The listing builds one solid part. Answer for the finished solid, in the listing's coordinates (mm). Give positions to 0.01 mm unless a question says otherwise; leave off trailing zeros. Answer as CSV lines item,"result". Start each with the question number.
(1) Each of these flat-tipped pins is pushed along its axis until it touches: pin 1 Ø10 at (x, y) = (89.5, -16.5) entering from -Z; pin 2 Ø1.6 at (x, z) = (107, 1) entering from -Y; pin 3 Ø1.5 at (x, z) = (129.5, 0.5) entering from -Y. Where does it stop, or does it pass through?
(2) Straight lines are drawn through the part: probe 1 along X at (y, z) = (-14, 2.8); probe 2 along Z at (x, y) = (13, -19.5); probe 3 along Y at (x, z) = (107.5, 0.85). For each, find the intervals that lie inside material, in ascending order.
(3) For a pull along Y with two mould halves and no side action, classify faces 1 (the face through (155.4, -14.46, 1.61)), 2 (the face through (164.332, -23.652, 1.61)), 3 (the face through (118.317, -15.718, 1.61)), 4 (the face through (142, -15, 3.175)) as pulls with the +Y half, pulls with the -Y half, needs draft (parallel to the pull), parting line crosses it, or undercut.
from build123d import *

# Parameters (mm, degrees)
F0_W     = 203.2
F0_H     = 38.1
F1_DEPTH = 3.175
F2_W     = 3.175
F2_H     = 4.445
F3_DEPTH = 25.4


# Not quite as in the source:
# - a feature names something its author has since deleted; it is built from what else it names


with BuildPart() as f1:
    # F0 (on Top) → F1 (new body)
    with BuildSketch(Plane.XY):
        with Locations((101.6, -19.05)):
            Rectangle(F0_W, F0_H)
    extrude(amount=F1_DEPTH)

    # F2 (on face) → F3 (cut)
    with BuildSketch(Plane.XY.offset(3.175)):
        with BuildLine():
            Line((0, -9.525), (0, -14.2875))
            ThreePointArc((0, -14.2875), (24.649723028, -4.4760985439), (50.8, 0))
            Line((50.8, 0), (0, 0))
            Line((0, 0), (0, -9.525))
        make_face()
        with Locations((103.1875, -35.8775)):
            Rectangle(F2_W, F2_H)
        with BuildLine():
            ThreePointArc((104.775, -30.48), (103.8450640303, -32.7250640303), (101.6, -33.655))
            Line((101.6, -33.655), (104.775, -33.655))
            Line((104.775, -33.655), (104.775, -30.48))
        make_face()
        with BuildLine():
            Line((104.775, -30.48), (101.6, -30.48))
            Line((101.6, -30.48), (101.6, -33.655))
            ThreePointArc((101.6, -33.655), (103.8450640303, -32.7250640303), (104.775, -30.48))
        make_face()
        with BuildLine():
            Line((101.6, -27.305), (101.6, -30.48))
            Line((101.6, -30.48), (104.775, -30.48))
            ThreePointArc((104.775, -30.48), (103.8450640303, -28.2349359697), (101.6, -27.305))
        make_face()
        with BuildLine():
            Line((98.4250000029, -30.4801362911), (101.6, -30.48))
            Line((101.6, -30.48), (101.6, -27.305))
            ThreePointArc((101.6, -27.305), (99.3548877841, -28.2349841564), (98.4250000029, -30.4801362911))
        make_face()
        with BuildLine():
            Line((101.6, -33.655), (101.6, -30.48))
            Line((101.6, -30.48), (98.4250000029, -30.4801362911))
            ThreePointArc((98.4250000029, -30.4801362911), (99.3549841564, -32.7251122159), (101.6, -33.655))
        make_face()
        with BuildLine():
            ThreePointArc((108.3690122037, -30.48), (106.4969075417, -31.9824905065), (104.775, -33.655))
            Line((104.775, -33.655), (104.775, -38.1))
            Line((104.775, -38.1), (184.15, -38.1))
            Line((184.15, -38.1), (193.675, -26.19375))
            ThreePointArc((193.675, -26.19375), (163.9135585822, -23.6655567526), (134.3847364187, -28.1581971794))
            ThreePointArc((134.3847364187, -28.1581971794), (121.0555708247, -25.7189035938), (108.3690122037, -30.48))
        make_face()
        with BuildLine():
            Line((101.6, -38.1), (101.6, -33.655))
            ThreePointArc((101.6, -33.655), (99.3549841564, -32.7251122159), (98.4250000029, -30.4801362911))
            Line((98.4250000029, -30.4801362911), (39.6036359929, -30.4826612755))
            ThreePointArc((39.6036359929, -30.4826612755), (18.2099329026, -26.2778753266), (0, -14.2875))
            Line((0, -14.2875), (0, -19.05))
            Line((0, -19.05), (0, -38.1))
            Line((0, -38.1), (101.6, -38.1))
        make_face()
        Polygon((203.2, 0), (184.15, 0), (203.2, -14.2875), align=None)
        Polygon((193.675, -26.19375), (184.15, -38.1), (203.2, -38.1), (203.2, -19.05), (203.2, -14.2875), align=None)
        with BuildLine():
            Line((108.3690122037, -30.48), (104.775, -30.48))
            Line((104.775, -30.48), (104.775, -33.655))
            ThreePointArc((104.775, -33.655), (106.4969075417, -31.9824905065), (108.3690122037, -30.48))
        make_face()
        with BuildLine():
            ThreePointArc((127.6218066335, -14.2875), (122.8593066335, -9.525), (118.0968066335, -14.2875))
            Line((118.0968066335, -14.2875), (127.6218066335, -14.2875))
        make_face()
        with BuildLine():
            Line((127.6218066335, -14.2875), (118.0968066335, -14.2875))
            ThreePointArc((118.0968066335, -14.2875), (122.8593066335, -19.05), (127.6218066335, -14.2875))
        make_face()
        with BuildLine():
            Line((176.8343066335, -14.2875), (183.1843066335, -14.2875))
            ThreePointArc((183.1843066335, -14.2875), (180.0093066335, -11.1125), (176.8343066335, -14.2875))
        make_face()
        with BuildLine():
            ThreePointArc((176.8343066335, -14.2875), (180.0093066335, -17.4625), (183.1843066335, -14.2875))
            Line((183.1843066335, -14.2875), (176.8343066335, -14.2875))
        make_face()
        with BuildLine():
            ThreePointArc((155.4030566335, -14.2875), (151.4343066335, -10.31875), (147.4655566335, -14.2875))
            Line((147.4655566335, -14.2875), (155.4030566335, -14.2875))
        make_face()
        with BuildLine():
            Line((155.4030566335, -14.2875), (147.4655566335, -14.2875))
            ThreePointArc((147.4655566335, -14.2875), (151.4343066335, -18.25625), (155.4030566335, -14.2875))
        make_face()
    extrude(amount=-F3_DEPTH, mode=Mode.SUBTRACT)

    # F8: sweep along a path in F5
    with BuildLine(Plane.XY.offset(1.5875)) as f8_path:
        Line((101.6, -30.48), (39.6036359929, -30.4826612755))
        ThreePointArc((39.6036359929, -30.4826612755), (18.2099329026, -26.2778753266), (0, -14.2875))
    # F7 (on offset) → F8 (sweep, cut)
    with BuildSketch(Plane.YZ.offset(101.6)):
        Polygon((-30.48, 3.1877), (-30.48, 1.5875), (-21.4048148322, 3.1877), align=None)
        Polygon((-21.4048148322, 3.1877), (-30.48, 1.5875), (0, 3.1877), align=None)
        Polygon((-21.4768401114, 0), (0, 0), (-30.48, 1.5875), align=None)
        Polygon((-4.1187478461, -3.0607), (-21.4768401114, 0), (-30.48, 0), (-30.48, -3.0607), align=None)
        Polygon((-30.48, 0), (-21.4768401114, 0), (-30.48, 1.5875), align=None)
        Polygon((-30.48, 6.2357), (-30.48, 3.1877), (-21.4048148322, 3.1877), (-4.1187478461, 6.2357), align=None)
    sweep(path=f8_path.line, mode=Mode.SUBTRACT)


solid = f1.part
Result set:
1,pin 1,"z = 0.6"
1,pin 2,"y = -30.48"
1,pin 3,"y = -26.58"
2,probe 1,"101.6 to 118.11, 127.61 to 147.48, 155.39 to 176.85, 183.17 to 202.82"
2,probe 2,"1.39 to 1.79"
2,probe 3,"-30.48 to 0"
3,face 1,"undercut"
3,face 2,"pulls with the -Y half"
3,face 3,"undercut"
3,face 4,"needs draft"
